```python
from build123d import *

# Parameters (mm, degrees)
F1_ANGLE    = 120
F2_T1_DEPTH = 60
F3_T2_ANGLE = 167.7805884334
F3_T4_ANGLE = 167.7805884334
F4_DEPTH    = 16
F5_R        = 2
F6_DEPTH    = 3.0010001
F5_W        = 60
F5_H        = 4
F7_DEPTH    = 3
F8_R        = 1.99999


# Not quite as in the source:
# - a fillet or chamfer that OpenCascade refuses, or shapes differently, is made with other operations: its cross-section is extruded or revolved along the edge and cut away or added
# - a fillet or chamfer is up to 0.001 mm smaller than in the source, because OpenCascade refuses the exact size


with BuildPart() as f1:
    # F0 (on Front) → F1 (revolve)
    with BuildSketch(Plane.XZ):
        Polygon((-33, 12), (-33, 0), (33, 0), (33, 12), (30, 12), (30, 3), (-30, 3), (-30, 12), align=None)
    revolve(axis=Axis((7.0132222027, 0, 30), (1, 0, 0)), revolution_arc=F1_ANGLE)

    # F2: chamfer of 3.9 x 6.7549981495 on 1 edges, made by hand

    # F2_s2 → F2_t1 (cut)
    with BuildSketch(Plane.YZ.offset(-30)):
        with BuildLine():
            Line((25.7683341911, 38.0618207012), (26.1129278328, 45.0763059136))
            Line((26.1129278328, 45.0763059136), (23.3826859022, 43.5))
            ThreePointArc((23.3826859022, 43.5), (24.7742012809, 40.7349406562), (25.7683341911, 38.0618207012))
        make_face()
    extrude(amount=F2_T1_DEPTH, mode=Mode.SUBTRACT)

    # F3: fillet of radius 5 on 2 edges, made by hand

    # F3_s1 → F3_t2 (revolve, cut)
    with BuildSketch(Plane(origin=(0, -11.1086546654, 4.9204270168), x_dir=(1, 0, 0), z_dir=(0, -0.9143225722, 0.4049867083))):
        with BuildLine():
            ThreePointArc((28, -2.5703228328), (31.5355339059, -1.1058567387), (33, 2.4296771672))
            Line((33, 2.4296771672), (33, -2.5703228328))
            Line((33, -2.5703228328), (28, -2.5703228328))
        make_face()
    revolve(axis=Axis((33, 0, 30), (1, 0, 0)), revolution_arc=F3_T2_ANGLE, mode=Mode.SUBTRACT)

    # F3_s3 → F3_t4 (revolve, cut)
    with BuildSketch(Plane(origin=(0, -11.1086546654, 4.9204270168), x_dir=(1, 0, 0), z_dir=(0, -0.9143225722, 0.4049867083))):
        with BuildLine():
            ThreePointArc((-33, 2.4296771672), (-31.5355339059, -1.1058567387), (-28, -2.5703228328))
            Line((-28, -2.5703228328), (-33, -2.5703228328))
            Line((-33, -2.5703228328), (-33, 2.4296771672))
        make_face()
    revolve(axis=Axis((-33, 0, 30), (1, 0, 0)), revolution_arc=F3_T4_ANGLE, mode=Mode.SUBTRACT)

    # F4 (add): a face of the model
    f4_faces = [f1.faces().sort_by_distance(p)[0] for p in [
        (0, 0, 2.8599348039),
    ]]
    extrude(f4_faces, amount=F4_DEPTH)

    # F5 (on face) → F6 (cut, through all)
    with BuildSketch(Plane.XY.offset(3)):
        with Locations((-8, -8)):
            Circle(F5_R)
        with Locations((8, -8)):
            Circle(F5_R)
    extrude(amount=-F6_DEPTH, mode=Mode.SUBTRACT)

    # F5 (on face) → F7 (join)
    with BuildSketch(Plane.XY.offset(3)):
        with Locations((0, -14)):
            Rectangle(F5_W, F5_H)
    extrude(amount=F7_DEPTH)

    # F8 (radius 2 in the source; OpenCascade refuses exactly that, so slightly less here)
    f8_edges = [f1.edges().sort_by_distance(p)[0] for p in [
        (0, -16, 6),
        (0, -12, 6),
    ]]
    fillet(f8_edges, radius=F8_R)


solid = f1.part
```
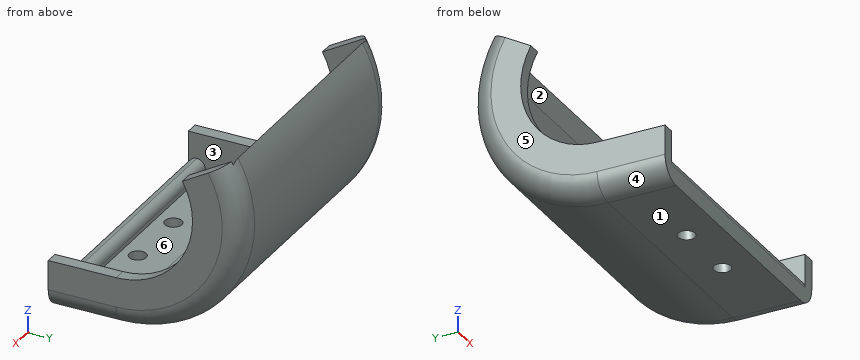
Geometry check sheet. Reference: the model listing, model coordinates, mm. Face numbers are marked on the shaded views. A direction names the side the tool comes from. Coordinates: 2 decimals unless noted, no trailing zeros. Write each loop counter-clockwise with the first axis right and the second up, starting at its lowest first coordinate (ties: lowest second). Pieces come first, ordered by that corner, then holes. Notation, with made-up numbers: M -16.75,2.5 L -10.75,2.5 A13 cw -10.75,9.5 Z; hole C -12,27 d10. An arc over 180 degrees is marked long. Answer as a JSON object with one key per item and string values.
1. Tool access check on the marked faces 5 and 6. Record the directions out of +Z, -Z, +X, -X, +Y, -Y that give a thin tool (end or side, any length) a straight path to the whole face; none if there is none.
Answers below:
{"face 5": "+Z, -Z, -X, +Y, -Y", "face 6": "+Z"}
2. Section check B-B, the plane y = -8. Enter the section's corners in (x, z), plus the area to 3 significant figures.
Answers below:
{"outline": "M -33,5 A5 ccw -28,0 L -10,0 L -10,3 L -30,3 L -30,12 L -33,12 Z; M -6,0 L 6,0 L 6,3 L -6,3 Z; M 10,0 L 28,0 A5 ccw 33,5 L 33,12 L 30,12 L 30,3 L 10,3 Z", "area": "217 mm²"}
3. Scan lines: L1, parallel to X at y = -13, z = 10; L2, parallel to Z at x = 28, y = -3; L3, parallel to Y at x = 28, z = 42. Record each from-to range of solid material in increasing order.
Answers below:
{"L1": "x = -33 to -30, 30 to 33", "L2": "z = 0 to 3", "L3": "y = 25.96 to 27.5"}
4. Draft check along X on the marked faces 1, 2, 3 and 4. Enter one of: released by +X, released by -X, zero draft, split by the parting line, or undercut.
Answers below:
{"face 1": "zero draft", "face 2": "undercut", "face 3": "undercut", "face 4": "released by -X"}
5. Go/stop test with flat-tipped pins: pin 1 Ø6 at (x, z) = (-18.5, 23) entering from +Y; pin 2 Ø1 at (x, y) = (23, 1) entering from +Z; pin 3 Ø6 at (x, y) = (-25.5, 7) entering from -Z. Record where each tip stops, or that it passes through.
Answers below:
{"pin 1": "stops at y = 29.73", "pin 2": "stops at z = 3.04", "pin 3": "stops at z = 0.27"}
